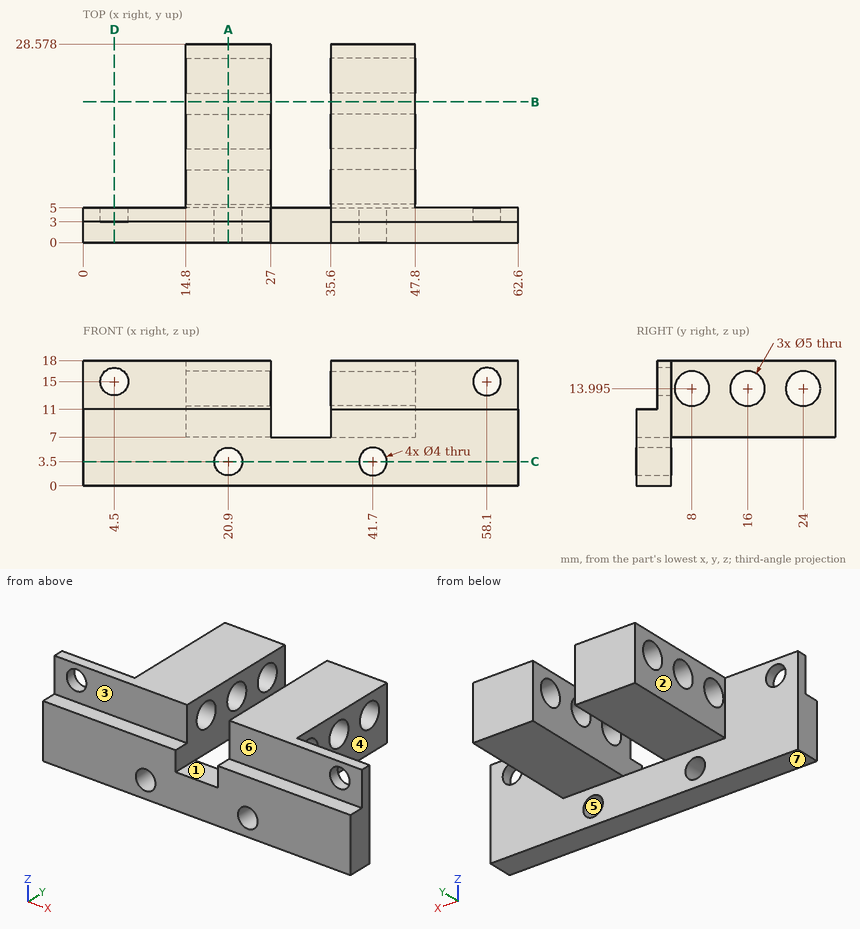
Here's the drawing with two shaded views (mm, measured from the low corner). I have some questions. A direction names the side the tool comes from. Coordinates: 2 decimals unless noted, no trailing zeros. Write each loop counter-clockwise with the first axis right and the second up, starting at its lowest first coordinate (ties: lowest second). Pieces come first, ordered by that corner, then holes. Notation, with made-up numbers: (33.5, 85.5) -> (45.5, 85.5) arc R14 cw to (45.5, 95.5) -> close; hole circle Ø10 at (12.5, 63). An arc over 180 degrees is marked (long way). One line per question, with ' | ' between items. Start each with the question number.
1. If we section it at B-B (y = 20.25): Please give me the cut outline in (x, z), and give its area (3 significant figures).
2. Thinking about a two-plate mould opening in Z: for the marked faces 5, 6 and 7, which applies, pulls with the +Z half, pulls with the -Z half, needs draft (parallel to the pull), parting line crosses it, or undercut?
3. For the marked faces 1, 2, 3 and 4, which set-ups out of +Z, -Z, +X, -X, +Y, -Y let a thin tool reach every point of the face, with its end or its side?
4. If we section it at C-C (z = 3.5): Please give me the cut outline in (x, y), and give its area (3 significant figures).
5. Please list where these lines run through material, in increasing order: line 1 along Y through (x, z) = (18.5, 14.25); line 2 along X through (y, z) = (3.35, 3.5); line 3 along Y through (x, z) = (39, 12).
6. If we section it at D-D (x = 4.5): Please give me the cut outline in (y, z), and give its area (3 significant figures).
7. If we section it at A-A (x = 20.9): Please give me the cut outline in (y, z) (3 decimals), and give its area (3 significant figures).
8. Will these pins go through, and if not, where does the flat tip stop? P1, Ø9, axis at y = 13.5, z = 10.5, coming from the -X side; P2, Ø4, axis at y = 16, z = 14, coming from the -X side; P3, Ø6, axis at y = 19, z = 5, coming from the +X side; P4, Ø0.9, axis at x = 51, y = 2, coming from the +Z side.
Return value:
1) outline: (14.8, 7) -> (27, 7) -> (27, 18) -> (14.8, 18) -> close; (35.6, 7) -> (47.8, 7) -> (47.8, 18) -> (35.6, 18) -> close | area: 268 mm²
2) face 5: undercut | face 6: needs draft | face 7: pulls with the -Z half
3) face 1: +Z, +Y, -Y | face 2: +Z, -Z, -X, +Y | face 3: +Z, +X, -X, -Y | face 4: +Z, -Z, +X, +Y
4) outline: (0, 0) -> (18.9, 0) -> (18.9, 5) -> (0, 5) -> close; (22.9, 0) -> (39.7, 0) -> (39.7, 5) -> (22.9, 5) -> close; (43.7, 0) -> (62.6, 0) -> (62.6, 5) -> (43.7, 5) -> close | area: 273 mm²
5) line 1: y = 3 to 5.51, 10.49 to 13.51, 18.49 to 21.51, 26.49 to 28.58 | line 2: x = 0 to 18.9, 22.9 to 39.7, 43.7 to 62.6 | line 3: y = 3 to 6.49, 9.51 to 14.49, 17.51 to 22.49, 25.51 to 28.58
6) outline: (0, 0) -> (5, 0) -> (5, 13) -> (3, 13) -> (3, 11) -> (0, 11) -> close; (3, 17) -> (5, 17) -> (5, 18) -> (3, 18) -> close | area: 61.0 mm²
7) outline: (0, 0) -> (5, 0) -> (5, 1.5) -> (0, 1.5) -> close; (0, 5.5) -> (5, 5.5) -> (5, 7) -> (28.578, 7) -> (28.578, 18) -> (3, 18) -> (3, 11) -> (0, 11) -> close; hole circle Ø5 at (8, 13.995); hole circle Ø5 at (16, 13.995); hole circle Ø5 at (24, 13.995) | area: 249 mm²
8) P1: stops at x = 14.8 | P2: passes through | P3: stops at x = 47.8 | P4: stops at z = 11
